Here's how the part is built. I have some questions about the finished solid (model axes, mm). A direction names the side the tool comes from. Round coordinates to 2 decimals unless told otherwise and drop trailing zeros. Order: outer loops, then holes, each group sorted by start corner. A loop starts at its lowest first (then second) coordinate and runs counter-clockwise, first axis right, second up. Notation, with made-up numbers: (-14, 7.25) - (23, 7.25) arc R21 ccw to (23, 25.25) - close; hole circle Ø9 at (-25.5, -16). An arc over 180 degrees is marked (long way). Answer as a JSON object with one key per item and string values.
```python
from build123d import *

# Parameters (mm, degrees)
SKETCH1_R               = 7.925
EXTRUDE1_DEPTH          = 25.4
SKETCH2_OUTSIDE_W       = 24.626
SKETCH2_OUTSIDE_H       = 24.626
SKETCH2_OUTSIDE_R       = 3.48
CUT_EXTRUDE1_DEPTH      = 12.75
SKETCH3_R               = 1.55
CUT_EXTRUDE2_DEPTH      = 8.925
CUT_EXTRUDE2_DEPTH_BACK = 8.925
SKETCH4_R               = 1.55
CUT_EXTRUDE3_DEPTH      = 8.925
CUT_EXTRUDE3_DEPTH_BACK = 8.925


with BuildPart() as part:
    # Sketch1 → Extrude1 (new body)
    with BuildSketch(Plane.XY):
        Circle(SKETCH1_R)
    extrude(amount=EXTRUDE1_DEPTH)

    # Sketch2 outside → Cut-Extrude1 (cut)
    with BuildSketch(Plane.XY):
        Rectangle(SKETCH2_OUTSIDE_W, SKETCH2_OUTSIDE_H)
        Circle(SKETCH2_OUTSIDE_R, mode=Mode.SUBTRACT)
    extrude(amount=CUT_EXTRUDE1_DEPTH, mode=Mode.SUBTRACT)

    # Sketch3 → Cut-Extrude2 (cut, two sides)
    with BuildSketch(Plane(origin=(0, 0, 0), x_dir=(1, 0, 0), z_dir=(0, 1, 0))) as cut_extrude2_sk:
        with Locations((0, -3.325)):
            Circle(SKETCH3_R)
    extrude(amount=CUT_EXTRUDE2_DEPTH, mode=Mode.SUBTRACT)
    extrude(cut_extrude2_sk.sketch, amount=-CUT_EXTRUDE2_DEPTH_BACK, mode=Mode.SUBTRACT)

    # Sketch4 → Cut-Extrude3 (cut, two sides)
    with BuildSketch(Plane(origin=(0, 0, 0), x_dir=(1, 0, 0), z_dir=(0, 1, 0))) as cut_extrude3_sk:
        with Locations((0, -19.05)):
            Circle(SKETCH4_R)
    extrude(amount=CUT_EXTRUDE3_DEPTH, mode=Mode.SUBTRACT)
    extrude(cut_extrude3_sk.sketch, amount=-CUT_EXTRUDE3_DEPTH_BACK, mode=Mode.SUBTRACT)


solid = part.part
```
1. For faces 1 (the face through (3.4, -1.7, 12.75)), 2 (the face through (3.66, -7.03, 18.99)), which set-ups out of +Z, -Z, +X, -X, +Y, -Y let a thin tool reach every point of the face, with its end or its side?
Responses:
{"face 1": "-Z", "face 2": "+Z, -Z"}
2. Imagine slicing it at A-A (x = 0). List the corners of the cut face in (y, z) for me (3 decimals), plus the area to 3 significant figures.
Responses:
{"outline": "(-7.925, 12.75) - (-3.48, 12.75) - (-3.48, 4.875) - (3.48, 4.875) - (3.48, 12.75) - (7.925, 12.75) - (7.925, 17.5) - (-7.925, 17.5) - close; (-7.925, 20.6) - (7.925, 20.6) - (7.925, 25.4) - (-7.925, 25.4) - close; (-3.48, 0) - (3.48, 0) - (3.48, 1.775) - (-3.48, 1.775) - close", "area": "219 mm2"}
3. Imagine slicing it at D-D (z = 13.25). List the corners of the cut face in (x, y) for me (3 decimals), plus the area to 3 significant figures.
Responses:
{"outline": "circle Ø15.85 at (0, 0)", "area": "197 mm2"}
4. If I drill on L1, parallel to Z at x = 0, y = -1.7 (3 decimals); L2, parallel to Z at x = 0, y = 6.75; L3, parallel to Z at x = 5.25, y = 4.5, over which ranges is the centre line in solid material (lowest first)? Write a range as [from, to].
Responses:
{"L1": "[0, 1.775], [4.875, 17.5], [20.6, 25.4]", "L2": "[12.75, 17.5], [20.6, 25.4]", "L3": "[12.75, 25.4]"}
5. For P1, Ø4, axis at y = -3, z = 5.5, coming from the +X side; P2, Ø2, axis at x = 5, y = -4.5, coming from the -Z side; P3, Ø2.5, axis at x = 0, z = 3.325, coming from the -Y side; P4, Ø6, axis at x = 5, z = 18, coming from the -Y side, each with a flat end and sliding along its axis, tell me the tip position at first contact or that it passes through.
Responses:
{"P1": "x = 3.33", "P2": "z = 12.75", "P3": "through", "P4": "y = -7.67"}
6. Imagine slicing it at C-C (y = 5.75). List the corners of the cut face in (x, z) for me, plus the area to 3 significant figures.
Responses:
{"outline": "(-5.45, 12.75) - (5.45, 12.75) - (5.45, 25.4) - (-5.45, 25.4) - close; hole circle Ø3.1 at (0, 19.05)", "area": "130 mm2"}
7. Imagine slicing it at B-B (z = 4.5). List the corners of the cut face in (x, y) for me.
Responses:
{"outline": "(-1.01, -3.33) - (-1.01, 3.33) arc R3.48 ccw to start; (1.01, -3.33) arc R3.48 ccw to (1.01, 3.33) - close"}
